```python
from build123d import *

# Parameters (mm, degrees)
SKETCH1_W           = 154.94
SKETCH1_H           = 40.64
BOSS_EXTRUDE1_DEPTH = 15.24
SKETCH2_W           = 30.988
SKETCH2_H           = 15.24
CUT_EXTRUDE1_DEPTH  = 161.904539401
SKETCH3_W           = 15.24
SKETCH3_H           = 8.466666666
SKETCH3_H_2         = 8.466666667
CUT_EXTRUDE2_DEPTH  = 161.904539401


with BuildPart() as part:
    # Sketch1 → Boss-Extrude1 (new body)
    with BuildSketch(Plane.XY):
        with Locations((77.47, 20.32)):
            Rectangle(SKETCH1_W, SKETCH1_H)
    extrude(amount=BOSS_EXTRUDE1_DEPTH)

    # Sketch2 → Cut-Extrude1 (cut, through all)
    with BuildSketch(Plane.XY.offset(15.24)):
        with Locations((15.494, 7.62)):
            Rectangle(SKETCH2_W, SKETCH2_H)
        with Locations((77.47, 7.62)):
            Rectangle(SKETCH2_W, SKETCH2_H)
        with Locations((139.446, 7.62)):
            Rectangle(SKETCH2_W, SKETCH2_H)
    extrude(amount=-CUT_EXTRUDE1_DEPTH, mode=Mode.SUBTRACT)

    # Sketch3 → Cut-Extrude2 (cut, through all)
    with BuildSketch(Plane.XY.offset(15.24)):
        with Locations((7.62, 27.94)):
            Rectangle(SKETCH3_W, SKETCH3_H)
        with Locations((147.32, 36.406666667)):
            Rectangle(SKETCH3_W, SKETCH3_H_2)
        with Locations((147.32, 19.473333334)):
            Rectangle(SKETCH3_W, SKETCH3_H_2)
    extrude(amount=-CUT_EXTRUDE2_DEPTH, mode=Mode.SUBTRACT)


solid = part.part
```
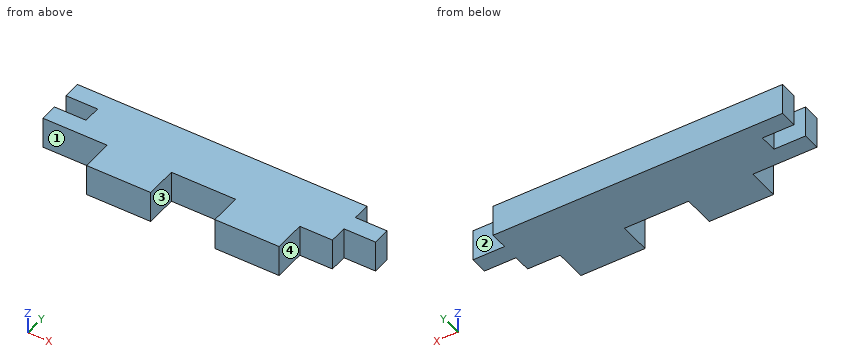
Here's how the part is built. I have some questions about the finished solid (model axes, mm). Face numbers are marked on the shaded views. A direction names the side the tool comes from. Give positions to 0.01 mm unless a question says otherwise; leave off trailing zeros. Loops run counter-clockwise (first coordinate to the right, second up) from the corner with the lowest first, then second, coordinate; pieces in that order, holes last. Notation, with made-up numbers: M -19.5,-39 L 35.5,-39 A27 cw 35.5,-15 Z; hole C -39.5,-36 d9. An arc over 180 degrees is marked long. Return JSON: item names as keys, results as strings.
Item 1: Imagine slicing it at A-A on y = 11.5. List the corners of the cut face in (x, z) for me, then the cut area to 3 significant figures.
A:
{"outline": "M 30.99,0 L 61.98,0 L 61.98,15.24 L 30.99,15.24 Z; M 92.96,0 L 123.95,0 L 123.95,15.24 L 92.96,15.24 Z", "area": "945 mm^2"}
Item 2: I'm going to push flat-ended pins straight in: pin 1 Ø3 at (x, y) = (96.5, 16) entering from -Z; pin 2 Ø4.5 at (x, z) = (146.5, 11.5) entering from -Y; pin 3 Ø2 at (y, z) = (22, 3) entering from +X; pin 4 Ø7 at (y, z) = (28, 7) entering from -X. Where does each tip first touch, or does it pass through?
A:
{"pin 1": "stops at z = 0", "pin 2": "stops at y = 23.71", "pin 3": "stops at x = 139.7", "pin 4": "stops at x = 15.24"}
Item 3: Please list where these lines run through material, in increasing order: line 1 (X direction, y = 4.5, z = 7); line 2 (Y direction, x = 12.5, z = 4.75); line 3 (Y direction, x = 15.5, z = 4.75).
A:
{"line 1": "x = 30.99 to 61.98, 92.96 to 123.95", "line 2": "y = 15.24 to 23.71, 32.17 to 40.64", "line 3": "y = 15.24 to 40.64"}
Item 4: On a 3-axis mill with a long thin cutter (end or side, diameter ignored), from which of +Z, -Z, +X, -X, +Y, -Y can I reach the whole of each face in a straight line? I mean the marked faces 1, 2, 3 and 4. Say none if no direction works.
A:
{"face 1": "+Z, -Z, -X, -Y", "face 2": "+Z, -Z, +X, +Y", "face 3": "+Z, -Z, -Y", "face 4": "+Z, -Z, +X, -Y"}
Item 5: Imagine slicing it at C-C on x = 133. List the corners of the cut face in (y, z) for me.
A:
{"outline": "M 15.24,0 L 40.64,0 L 40.64,15.24 L 15.24,15.24 Z"}
Item 6: Imagine slicing it at B-B on z = 12.5. List the corners of the cut face in (x, y) for me.
A:
{"outline": "M 0,15.24 L 30.99,15.24 L 30.99,0 L 61.98,0 L 61.98,15.24 L 92.96,15.24 L 92.96,0 L 123.95,0 L 123.95,15.24 L 139.7,15.24 L 139.7,23.71 L 154.94,23.71 L 154.94,32.17 L 139.7,32.17 L 139.7,40.64 L 0,40.64 L 0,32.17 L 15.24,32.17 L 15.24,23.71 L 0,23.71 Z"}
Item 7: Imagine slicing it at D-D on y = 35. List the corners of the cut face in (x, z) for me, then the cut area to 3 significant figures.
A:
{"outline": "M 0,0 L 139.7,0 L 139.7,15.24 L 0,15.24 Z", "area": "2,130 mm^2"}
